Here's how the part is built. I have some questions about the finished solid (model axes, mm). Face numbers are marked on the shaded views. A direction names the side the tool comes from. Round coordinates to 2 decimals unless told otherwise and drop trailing zeros. Write each loop counter-clockwise with the first axis right and the second up, starting at its lowest first coordinate (ties: lowest second). Pieces come first, ordered by that corner, then holes. Notation, with made-up numbers: (60, -1.5) - (117, -1.5) arc R15 ccw to (117, 10.5) - close; hole circle Ø8 at (73.25, 69.5). An arc over 180 degrees is marked (long way). One line per item, written item: value. Start each with the question number.
Item 1: Imagine slicing it at A-A, the plane y = -0.85. Count the separate pieces of the cut face and the enclosed holes in it, then the cut area to 3 significant figures.
Item 2: Thinking about a two-plate mould opening in Z: for the marked faces 3, 4 and 5, which applies, released by +Z, released by -Z, zero draft, split by the parting line, or undercut?
Item 3: If I drill on line 1 (Z direction, x = -2, y = -0.45); line 2 (Y direction, x = -2, z = 12); line 3 (X direction, y = 2, z = 13.25), over which ranges is the centre line in solid material (lowest first)?
Item 4: For the marked faces 1 and 2, which set-ups out of +Z, -Z, +X, -X, +Y, -Y let a thin tool reach every point of the face, with its end or its side?
Item 5: For P1, Ø3, axis at x = -0.5, z = 11.5, coming from the +Y side; P2, Ø1.5, axis at x = 1.5, z = 7, coming from the +Y side, each with a flat end and sliding along its axis, tell me the tip position at first contact or that it passes through.
Item 6: Imagine slicing it at B-B, the plane z = 3.5. Please give me the cut outline in (x, y), then the cut area to 3 significant figures.
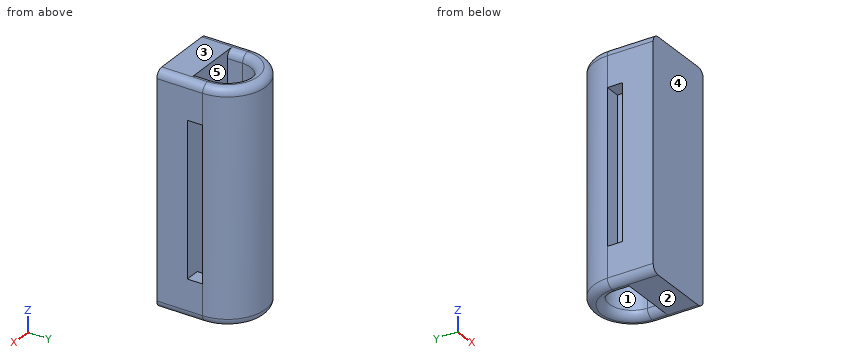
```python
from build123d import *

# Parameters (mm, degrees)
DODANIE_WYCI_GNI_CIE2_DEPTH = 15
SZKIC3_W                    = 1
SZKIC3_H                    = 2.5
DODANIE_WYCI_GNI_CIE3_DEPTH = 3
SZKIC4_W                    = 1
SZKIC4_H                    = 2
DODANIE_WYCI_GNI_CIE4_DEPTH = 10
SZKIC6_W                    = 15
SZKIC6_H                    = 2
DODANIE_WYCI_GNI_CIE5_DEPTH = 3
ZAOKR_GLENIE1_R             = 0.5


with BuildPart() as part:
    # Szkic1 → Dodanie-wyciągnięcie2 (new body)
    with BuildSketch(Plane.XY):
        with BuildLine():
            ThreePointArc((-2.5, 0), (0, 2.5), (2.5, 0))
            Line((2.5, 0), (1.5, 0))
            ThreePointArc((1.5, 0), (0, 1.5), (-1.5, 0))
            Line((-1.5, 0), (-2.5, 0))
        make_face()
    extrude(amount=DODANIE_WYCI_GNI_CIE2_DEPTH)

    # Szkic3 → Dodanie-wyciągnięcie3 (add)
    with BuildSketch(Plane.XZ):
        with Locations((-2, 13.75)):
            Rectangle(SZKIC3_W, SZKIC3_H)
        with Locations((2, 13.75)):
            Rectangle(SZKIC3_W, SZKIC3_H)
        with Locations((2, 1.25)):
            Rectangle(SZKIC3_W, SZKIC3_H)
        with Locations((-2, 1.25)):
            Rectangle(SZKIC3_W, SZKIC3_H)
    extrude(amount=DODANIE_WYCI_GNI_CIE3_DEPTH)

    # Szkic4 → Dodanie-wyciągnięcie4 (add)
    with BuildSketch(Plane(origin=(0, 0, 12.5), x_dir=(-1, 0, 0), z_dir=(0, 0, -1))):
        with Locations((2, -2)):
            Rectangle(SZKIC4_W, SZKIC4_H)
        with Locations((-2, -2)):
            Rectangle(SZKIC4_W, SZKIC4_H)
    extrude(amount=DODANIE_WYCI_GNI_CIE4_DEPTH)

    # Szkic6 → Dodanie-wyciągnięcie5 (add)
    with BuildSketch(Plane(origin=(-1.5, 0, 0), x_dir=(0, 0, -1), z_dir=(1, 0, 0))):
        with Locations((-7.5, -2)):
            Rectangle(SZKIC6_W, SZKIC6_H)
    extrude(amount=DODANIE_WYCI_GNI_CIE5_DEPTH)

    # Zaokrąglenie1
    zaokr_glenie1_edges = [part.edges().sort_by_distance(p)[0] for p in [
        (0, 1.5, 15),
        (-2.5, -1.5, 15),
        (2.5, -1.5, 15),
        (2.5, -1.5, 0),
        (-2.5, -1.5, 0),
        (0, 2.5, 15),
        (0, 1.5, 0),
        (0, 2.5, 0),
        (1.5, -0.5, 0),
        (1.5, -0.5, 15),
        (-1.5, -0.5, 15),
        (-1.5, -0.5, 0),
    ]]
    fillet(zaokr_glenie1_edges, radius=ZAOKR_GLENIE1_R - 0.0001)  # a hair under: the kernel refuses the full size


solid = part.part
```
Values follow:
1. separate pieces: 4
1. enclosed holes: 0
1. area: 9.57 mm^2
2. face 3: released by +Z
2. face 4: zero draft
2. face 5: undercut
3. line 1: z = 0 to 2.5, 12.5 to 15
3. line 2: y = -3 to -1, 0 to 1.5
3. line 3: x = -1.5 to 1.5
4. face 1: +Z, -Z
4. face 2: -Z, +X, -X, +Y, -Y
5. P1: stops at y = 2.5
5. P2: stops at y = 2.38
6. outline: (-2.5, -3) - (2.5, -3) - (2.5, -1) - (-2.5, -1) - close; (-2.5, 0) - (-1.5, 0) arc R1.5 cw to (1.5, 0) - (2.5, 0) arc R2.5 ccw to start
6. area: 16.3 mm^2
